Solid Edge part; units mm, degrees
sketch "Sketch1" plane through (0, 0, 0) normal (0, -1, 0) x (1, 0, 0)
  line L0 (-70.35, 58.75) -> (-70.35, -58.75)
  line L1 (-70.35, -58.75) -> (70.35, -58.75)
  line L2 (70.35, -58.75) -> (70.35, 58.75)
  line L3 (70.35, 58.75) -> (-70.35, 58.75)
extrude "Protrusion1" add sketch "Sketch1" against normal blind 150
sketch "Sketch2" plane through (70.35, 75, 0) normal (1, 0, 0) x (0, 1, 0)
  line L0 (75, 58.75) -> (75, 52.25)
  line L1 (75, 52.25) -> (55, 52.25)
  line L2 (55, 52.25) -> (45, 58.75)
  line L3 (45, 58.75) -> (75, 58.75)
  dimension "D1" = 45
  dimension "D2" = 75
  dimension "D3" = 75
extrude "ExtrudedCutout_1" cut sketch "Sketch2" against normal blind 172.2631
fillet "Round_2" radius 15 18 edges at (70.35, 60, 58.75) (0, 120, 58.75) (-70.35, 60, 58.75) (0, 0, 58.75) (-70.35, 0, 0) (0, 0, -58.75) (70.35, 0, 0) (70.35, 150, -3.25) (70.35, 140, 52.25) (70.35, 125, 55.5) (70.35, 75, -58.75) (-70.35, 125, 55.5) (-70.35, 140, 52.25) (-70.35, 150, -3.25) (-70.35, 75, -58.75) (0, 150, -58.75) (0, 150, 52.25) (0, 130, 52.25)
Work out the finished part from the listing and answer in its coordinate system (mm). A direction names the side the tool comes from. Give positions to 0.01 mm unless a question says otherwise; leave off trailing zeros. Order: outer loops, then holes, each group sorted by start corner. A loop starts at its lowest first (then second) coordinate and runs counter-clockwise, first axis right, second up. Notation, with made-up numbers: M 65.5,43.25 L 93.5,43.25 A12 cw 93.5,63.25 Z; hole C 8.25,53.5 d6. An arc over 180 degrees is marked long. Return JSON: item names as keys, results as strings.
Q1. Find the intervals of material crossed by line 1 along Y through (x, z) = (64, -18); line 2 along Z through (x, y) = (64, 17.5); line 3 along Z through (x, y) = (64, 13.5), in increasing order. Write a range as [from, to].
Answer below:
{"line 1": "y = [2.75, 147.25]", "line 2": "z = [-56, 56]", "line 3": "z = [-55.91, 55.91]"}
Q2. Find section B-B, the plane x = 59. Write down the section's boundary in (y, z).
Answer below:
{"outline": "M 0.45,-43.75 A14.55 ccw 15,-58.3 L 135,-58.3 A14.55 ccw 149.55,-43.75 L 149.55,37.25 A14.55 ccw 135,51.8 L 134.45,51.8 A15.45 cw 126.03,54.3 L 123.48,55.95 A14.55 ccw 115.55,58.3 L 15,58.3 A14.55 ccw 0.45,43.75 Z"}
Q3. Find section A-A, the plane x = -45. Write down the section's boundary in (y, z), and give its area (3 significant figures).
Answer below:
{"outline": "M 0,-43.75 A15 ccw 15,-58.75 L 135,-58.75 A15 ccw 150,-43.75 L 150,37.25 A15 ccw 135,52.25 L 134.45,52.25 A15 cw 126.27,54.67 L 123.73,56.33 A15 ccw 115.55,58.75 L 15,58.75 A15 ccw 0,43.75 Z", "area": "17,300 mm^2"}
Q4. This flat-tipped pin is pushed along its axis until it touches: pin 1 (6 mm diameter, centred on x = -56, z = 24.5, fed in from -Y). Where does it stop, or does it pass through?
Answer below:
{"pin 1": "stops at y = 0"}
Q5. Which of the six approach directions +Z, -Z, +X, -X, +Y, -Y give full straight-line access (tool end or side, diameter ignored) to faces 1 (the face through (-1, 74, -58.75)), 2 (the face through (66.07, 134.72, 47.74))?
Answer below:
{"face 1": "-Z, +X, -X, +Y, -Y", "face 2": "+Z, +X, +Y"}
